```python
from build123d import *

# Parameters (mm, degrees)
REVOLVE3_ANGLE           = 35
REVOLVE3_OTHER_WAY_ANGLE = 35
CIRPATTERN1_COUNT        = 6
SKETCH8_OUTSIDE_W        = 42.448
SKETCH8_OUTSIDE_H        = 43.096
SKETCH8_OUTSIDE_R        = 14
CUT_EXTRUDE1_DEPTH       = 24.946705857


with BuildPart() as part:
    # Sketch1 → Revolve1 (revolve)
    with BuildSketch(Plane.XY, mode=Mode.PRIVATE) as revolve1_sk:
        with BuildLine():
            Line((-10, 9), (-1.75, 9))
            ThreePointArc((-1.75, 9), (-1.573223305, 8.926776695), (-1.5, 8.75))
            Line((-1.5, 8.75), (-1.5, 0))
            Line((-1.5, 0), (-3, 0))
            Line((-3, 0), (-3, 7.75))
            Line((-3, 7.75), (-10, 7.75))
            Line((-10, 7.75), (-10, 9))
        make_face()
    revolve(revolve1_sk.sketch.rotate(Axis((0, 0, 0), (-1, 0, 0)), 90), axis=Axis((0, 0, 0), (-1, 0, 0)))


with BuildPart() as body_2:
    # Sketch6 → Revolve3 (revolve)
    with BuildSketch(Plane(origin=(-0.750692152, 0.026214748, 2.031649583), x_dir=(-0.9380241231891524, -0.004471483741222242, -0.3465411233149307), z_dir=(0.34656997030213393, -0.01210249004568391, -0.9379460461132464))):
        Polygon((5.267365496, 15.988922273), (4.268057854, 15.951716943), (4.565700491, 7.957255807), (5.565008133, 7.994461136), align=None)
    revolve(axis=Axis((-9.5, 5.745, -1.275), (0.4834449794238033, -0.8545819713199232, 0.18965918423549216)), revolution_arc=REVOLVE3_ANGLE)

    # Sketch6 → Revolve3 other way (revolve)
    with BuildSketch(Plane(origin=(-0.750692152, 0.026214748, 2.031649583), x_dir=(-0.9380241231891524, -0.004471483741222242, -0.3465411233149307), z_dir=(0.34656997030213393, -0.01210249004568391, -0.9379460461132464))):
        Polygon((5.267365496, 15.988922273), (4.268057854, 15.951716943), (4.565700491, 7.957255807), (5.565008133, 7.994461136), align=None)
    revolve(axis=Axis((-9.5, 5.745, -1.275), (-0.4834449794238033, 0.8545819713199232, -0.18965918423549216)), revolution_arc=REVOLVE3_OTHER_WAY_ANGLE)


with BuildPart() as cirpattern1_1:
    # CirPattern1: pattern copy
    add(body_2.part.rotate(Axis((0, 0, 0), (1, 0, 0)), 1 * 360 / CIRPATTERN1_COUNT))


with BuildPart() as cirpattern1_2:
    # CirPattern1: pattern copy
    add(body_2.part.rotate(Axis((0, 0, 0), (1, 0, 0)), 2 * 360 / CIRPATTERN1_COUNT))


with BuildPart() as cirpattern1_3:
    # CirPattern1: pattern copy
    add(body_2.part.rotate(Axis((0, 0, 0), (1, 0, 0)), 3 * 360 / CIRPATTERN1_COUNT))


with BuildPart() as cirpattern1_4:
    # CirPattern1: pattern copy
    add(body_2.part.rotate(Axis((0, 0, 0), (1, 0, 0)), 4 * 360 / CIRPATTERN1_COUNT))


with BuildPart() as cirpattern1_5:
    # CirPattern1: pattern copy
    add(body_2.part.rotate(Axis((0, 0, 0), (1, 0, 0)), 5 * 360 / CIRPATTERN1_COUNT))


with BuildPart() as cirpattern1_3_1:
    add(cirpattern1_3.part)

    # Combine1: union CirPattern1_5, CirPattern1_2, part, CirPattern1_4, body 2, CirPattern1_1
    add(cirpattern1_5.part)
    add(cirpattern1_2.part)
    add(part.part)
    add(cirpattern1_4.part)
    add(body_2.part)
    add(cirpattern1_1.part)

    # Sketch8 outside → Cut-Extrude1 (cut, through all)
    with BuildSketch(Plane(origin=(-1.5, 0, 0), x_dir=(0, 0, -1), z_dir=(1, 0, 0))):
        Rectangle(SKETCH8_OUTSIDE_W, SKETCH8_OUTSIDE_H)
        Circle(SKETCH8_OUTSIDE_R, mode=Mode.SUBTRACT)
    extrude(amount=-CUT_EXTRUDE1_DEPTH, mode=Mode.SUBTRACT)


solid = cirpattern1_3_1.part
```
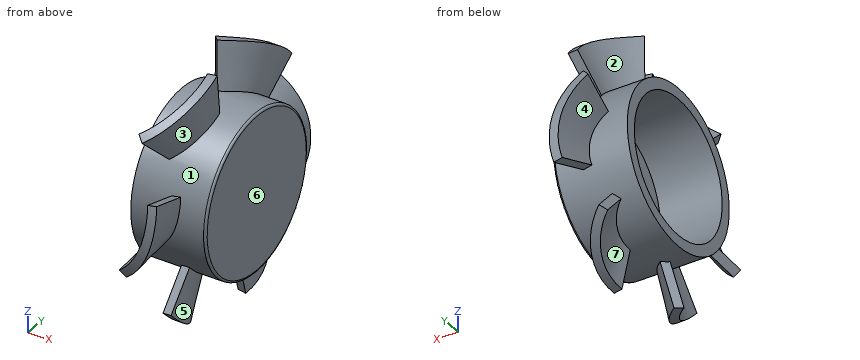
Can you work these out from the model? Positions are in its coordinate system, mm. Face numbers are marked on the shaded views. A direction names the side the tool comes from. Round coordinates to 2 decimals unless told otherwise and drop trailing zeros. Loops run counter-clockwise (first coordinate to the right, second up) from the corner with the lowest first, then second, coordinate; pieces in that order, holes last.
Item 1: Which directions (+Z, -Z, +X, -X, +Y, -Y) give clear straight access to the entire face, cutting with the end or side of a thin tool? Please do the marked faces 1, 2 and 3.
Item 2: Suppose I cut it at B-B, the plane x = -2.5. Write out the boundary of the cut face in (y, z).
Item 3: Please list where these lines run through material, in increasing order: L1, parallel to Y at x = -8, z = 0; L2, parallel to X at y = -7, z = -1.5; L3, parallel to Z at x = -4, y = 3.25.
Item 4: Will these pins go through, and if not, where does the flat tip stop? pin 1 Ø4.5 at (y, z) = (0.5, 0.5) entering from -X; pin 2 Ø3 at (x, y) = (-4.5, -9) entering from +Z; pin 3 Ø4 at (y, z) = (-4.5, -8) entering from -X; pin 4 Ø1 at (y, z) = (8.5, 4.5) entering from +X.
Item 5: If we mould it in two halves opening along Y, with no side actions, what happens to the marked faces 4, 5, 6 and 7? For each: +Y half, -Y half, draft (parallel to the pull), parting line (faces both ways), or undercut.
Item 6: Suppose I cut it at A-A, the plane y = 0. Write out the boundary of the cut face in (x, z).
Reported:
1. face 1: none
1. face 2: -X
1. face 3: +X
2. outline: circle Ø18 at (0, 0)
3. L1: y = -9 to -7.75, 7.75 to 9
3. L2: x = -3 to -1.5
3. L3: z = -8.39 to -7.04, 7.04 to 8.39
4. pin 1: stops at x = -3
4. pin 2: stops at z = 11.78
4. pin 3: stops at x = -10
4. pin 4: passes through
5. face 4: +Y half
5. face 5: undercut
5. face 6: draft
5. face 7: undercut
6. outline: (-10, -9) - (-1.75, -9) arc R0.25 ccw to (-1.5, -8.75) - (-1.5, 8.75) arc R0.25 ccw to (-1.75, 9) - (-10, 9) - (-10, 7.75) - (-3, 7.75) - (-3, -7.75) - (-10, -7.75) - close
